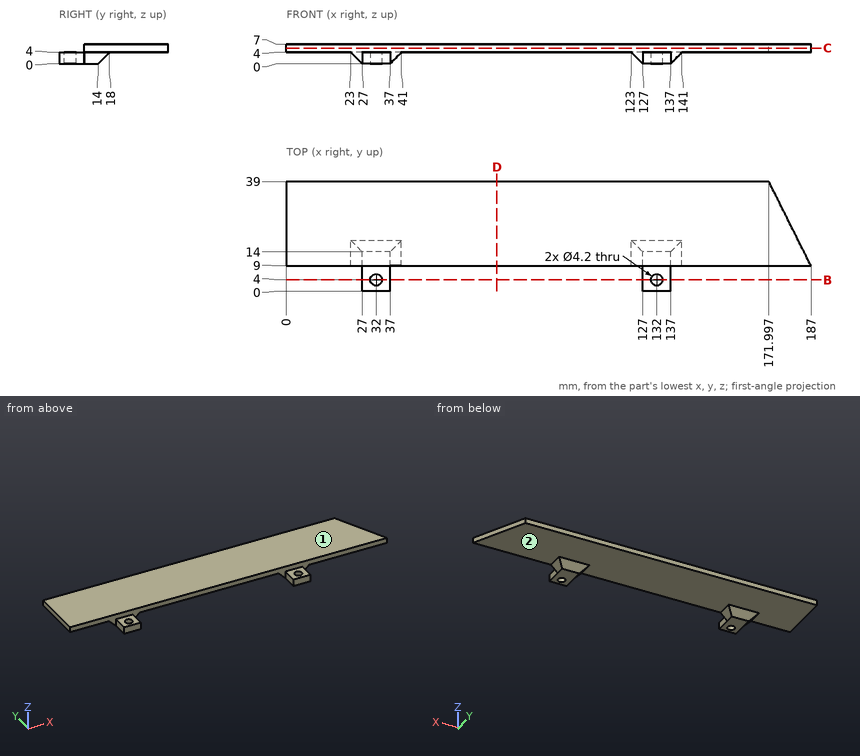
Input: dimensioned drawing with shaded views. Units: mm. Origin: part minimum x, y, z. A direction names the side the tool comes from. Round coordinates to 2 decimals unless told otherwise and drop trailing zeros. Loops run counter-clockwise (first coordinate to the right, second up) from the corner with the lowest first, then second, coordinate; pieces in that order, holes last. Notation, with made-up numbers: M 38.5,83.25 L 65.5,83.25 A24 ccw 65.5,110.25 Z; hole C 62,83 d1. An arc over 180 degrees is marked long. Answer in a Markdown table with one row per item. Add a question column.
1. Section C-C (z = 5.5). Output: boundary loops of the cut face in (x, y), and give its area (4 significant figures).
2. Section B-B (y = 4). Output: boundary loops of the cut face in (x, z).
3. Contact query for flat-ended pins moving along their axis: pin 1 (3 mm diameter, centred on y = 5, z = 1, fed in from -X); pin 2 (3 mm diameter, centred on x = 138.5, z = 6, fed in from -Y); pin 3 (4.5 mm diameter, centred on x = 34, y = 3.5, fed in from +Z); pin 4 (1 mm diameter, centred on y = 16.5, z = 1.5, fed in from +X). Output: stop coordinate, or through.
4. Set-up query: the marked faces 1 and 2. Return all of +Z, -Z, +X, -X, +Y, -Y with unobstructed straight access to the full face (end or side cutting, diameter ignored); none if empty.
5. Ray query, probe 1 along Z at (x, y) = (151, 35); probe 2 along Y at (x, z) = (47, 5.5); probe 3 along Y at (x, z) = (132, 1.3). Return the intervals inside material, ascending.
6. Section D-D (x = 75). Output: boundary loops of the cut face in (y, z), and give its area (3 significant figures).
Values follow:
| question | item | result |
|---|---|---|
| 1 | outline | M 0,9 L 187,9 L 172,39 L 0,39 Z |
| 1 | area | 5,385 mm^2 |
| 2 | outline | M 27,0 L 29.9,0 L 29.9,4 L 27,4 Z; M 34.1,0 L 37,0 L 37,4 L 34.1,4 Z; M 127,0 L 129.9,0 L 129.9,4 L 127,4 Z; M 134.1,0 L 137,0 L 137,4 L 134.1,4 Z |
| 3 | pin 1 | x = 27 |
| 3 | pin 2 | y = 9 |
| 3 | pin 3 | z = 4 |
| 3 | pin 4 | through |
| 4 | face 1 | +Z, +X, -X, +Y, -Y |
| 4 | face 2 | -Z, +Y |
| 5 | probe 1 | 4 to 7 |
| 5 | probe 2 | 9 to 39 |
| 5 | probe 3 | 0 to 1.9, 6.1 to 15.3 |
| 6 | outline | M 9,4 L 39,4 L 39,7 L 9,7 Z |
| 6 | area | 90.0 mm^2 |
